Part model, mm, in its own coordinate system. A direction names the side the tool comes from. Coordinates: 2 decimals unless noted, no trailing zeros. One line per question, with ' | ' between items. Start each with the question number.
Autodesk Fusion 360 part; units mm, degrees
sketch "Sketch1" plane through (0, 0, 0) normal (0, 1, 0) x (1, 0, 0)
  circle A0 centre (0, 0) radius 57.5
  line L0 (36, -36) -> (-36, -36) construction
  line L1 (-36, -36) -> (-36, 36) construction
  line L2 (-36, 36) -> (36, 36) construction
  line L3 (36, 36) -> (36, -36) construction
  line L4 (36, -36) -> (-36, 36) construction
  line L5 (-36, -36) -> (36, 36) construction
  circle A1 centre (0, 0) radius 43
  circle A2 centre (-36, 36) radius 2
  circle A3 centre (36, 36) radius 2
  circle A4 centre (36, -36) radius 2
  circle A5 centre (-36, -36) radius 2
  circle A6 centre (-36, -36) radius 2.875
  circle A7 centre (36, -36) radius 2.875
  circle A8 centre (36, 36) radius 2.875
  circle A9 centre (-36, 36) radius 2.875
  line L6 (52.5, 40.4773) -> (52.5, -51.7956) construction
  line L7 (67.5556, 30.3847) -> (52.5, 30.3847)
  line L8 (52.5, 30.3847) -> (52.5, -29.8632)
  line L9 (-46.2969, -51.75) -> (48.3967, -51.75)
  arc A10 (-25.0637, -51.75) -> (25.0637, -51.75) centre (0, 0) ccw
  dimension "d1" = 115
  dimension "d2" = 72
  dimension "d3" = 72
  dimension "d4" = 86
  dimension "d5" = 4
  dimension "d6" = 4
  dimension "d7" = 4
  dimension "d8" = 4
  dimension "d9" = 5.75
  dimension "d10" = 5.75
  dimension "d11" = 5.75
  dimension "d12" = 5.75
  dimension "d54" = 52.5
  dimension "d58" = 51.75
extrude "Extrude1" add sketch "Sketch1" along normal blind 4 contours A0 L9 A10 | A0 L8 L9 | A0 L8
extrude "Extrude3" add sketch "Sketch1" along normal blind 2 contours A1
sketch "Sketch2" plane through (0, 2, 0) normal (0, 1, 0) x (-1, 0, 0)
  circle A0 centre (0, 0) radius 43
  circle A1 centre (0, 0) radius 35 construction
  circle A2 centre (0, 0) radius 27.5 construction
  circle A3 centre (0, 0) radius 20 construction
  circle A4 centre (0, 0) radius 12.5 construction
  circle A5 centre (0, 0) radius 7.5 construction
  circle A6 centre (-0.2536, -34.9991) radius 3.5
  circle A7 centre (10.5741, -33.3645) radius 3.5
  circle A8 centre (20.3668, -28.4639) radius 3.5
  circle A9 centre (28.1658, -20.7771) radius 3.5
  circle A10 centre (33.2077, -11.0565) radius 3.5
  circle A11 centre (34.9991, -0.2536) radius 3.5
  circle A12 centre (33.3645, 10.5741) radius 3.5
  circle A13 centre (28.4639, 20.3668) radius 3.5
  circle A14 centre (20.7771, 28.1658) radius 3.5
  circle A15 centre (11.0565, 33.2077) radius 3.5
  circle A16 centre (0.2536, 34.9991) radius 3.5
  circle A17 centre (-10.5741, 33.3645) radius 3.5
  circle A18 centre (-20.3668, 28.4639) radius 3.5
  circle A19 centre (-28.1658, 20.7771) radius 3.5
  circle A20 centre (-33.2077, 11.0565) radius 3.5
  circle A21 centre (-34.9991, 0.2536) radius 3.5
  circle A22 centre (-33.3645, -10.5741) radius 3.5
  circle A23 centre (-28.4639, -20.3668) radius 3.5
  circle A24 centre (-20.7771, -28.1658) radius 3.5
  circle A25 centre (-11.0565, -33.2077) radius 3.5
  circle A26 centre (4.2963, -27.1623) radius 3.5
  circle A27 centre (12.4797, -24.5053) radius 3.5
  circle A28 centre (19.4414, -19.4495) radius 3.5
  circle A29 centre (24.5001, -12.4898) radius 3.5
  circle A30 centre (27.1605, -4.3076) radius 3.5
  circle A31 centre (27.1623, 4.2963) radius 3.5
  circle A32 centre (24.5053, 12.4797) radius 3.5
  circle A33 centre (19.4495, 19.4414) radius 3.5
  circle A34 centre (12.4898, 24.5001) radius 3.5
  circle A35 centre (4.3076, 27.1605) radius 3.5
  circle A36 centre (-4.2963, 27.1623) radius 3.5
  circle A37 centre (-12.4797, 24.5053) radius 3.5
  circle A38 centre (-19.4414, 19.4495) radius 3.5
  circle A39 centre (-24.5001, 12.4898) radius 3.5
  circle A40 centre (-27.1605, 4.3076) radius 3.5
  circle A41 centre (-27.1623, -4.2963) radius 3.5
  circle A42 centre (-24.5053, -12.4797) radius 3.5
  circle A43 centre (-19.4495, -19.4414) radius 3.5
  circle A44 centre (-12.4898, -24.5001) radius 3.5
  circle A45 centre (-4.3076, -27.1605) radius 3.5
  circle A46 centre (0.1335, -19.9996) radius 3.5
  circle A47 centre (11.8634, -16.1015) radius 3.5
  circle A48 centre (19.0619, -6.0533) radius 3.5
  circle A49 centre (18.9795, 6.3071) radius 3.5
  circle A50 centre (11.6475, 16.2584) radius 3.5
  circle A51 centre (-0.1335, 19.9996) radius 3.5
  circle A52 centre (-11.8634, 16.1015) radius 3.5
  circle A53 centre (-19.0619, 6.0533) radius 3.5
  circle A54 centre (-18.9795, -6.3071) radius 3.5
  circle A55 centre (-11.6475, -16.2584) radius 3.5
  circle A56 centre (4.3124, -11.7326) radius 3.5
  circle A57 centre (10.3851, -6.957) radius 3.5
  circle A58 centre (12.4909, 0.4758) radius 3.5
  circle A59 centre (9.8257, 7.7269) radius 3.5
  circle A60 centre (3.4074, 12.0266) radius 3.5
  circle A61 centre (-4.3124, 11.7326) radius 3.5
  circle A62 centre (-10.3851, 6.957) radius 3.5
  circle A63 centre (-12.4909, -0.4758) radius 3.5
  circle A64 centre (-9.8257, -7.7269) radius 3.5
  circle A65 centre (-3.4074, -12.0266) radius 3.5
  circle A66 centre (-0.0342, -5.0724) radius 2.5
  circle A67 centre (4.8135, -1.6) radius 2.5
  circle A68 centre (3.0092, 4.0835) radius 2.5
  circle A69 centre (-2.9538, 4.1238) radius 2.5
  circle A70 centre (-4.8347, -1.5349) radius 2.5
  dimension "d19" = 70
  dimension "d20" = 55
  dimension "d21" = 40
  dimension "d22" = 25
  dimension "d23" = 15
  dimension "d24" = 7
  dimension "d28" = 360
  dimension "d29" = 7
  dimension "d31" = 360
  dimension "d32" = 7
  dimension "d34" = 360
  dimension "d35" = 7
  dimension "d43" = 360
  dimension "d45" = 5
  dimension "d47" = 360
extrude "Extrude4" cut sketch "Sketch2" against normal up to surface (2 mm away) contours A6
extrude "Extrude5" cut sketch "Sketch2" against normal up to surface (2 mm away) contours A7 | A8 | A9 | A10 | A11 | A12 | A13 | A14 | A15 | A16 | A17 | A18 | A19 | A20 | A21 | A22 | A23 | A24 | A25 | A26 | A27 | A28 | A29 | A30 | A31 | A32 | A33 | A34 | A35 | A36 | A37 | A38 | A39 | A40 | A41 | A42 | A43 | A44 | A45 | A46 | A47 | A48 | A49 | A50 | A51 | A52 | A53 | A54 | A55 | A56 | A57 | A58 | A59 | A60 | A61 | A62 | A63 | A64 | A65 | A66 | A67 | A68 | A69 | A70
extrude "Extrude6" add sketch "Sketch1" against normal blind 2 from surface at 4 contours A6 | A7 | A8 | A9
chamfer "Chamfer1" distance 3 angle 45 1 edges at (-53.6088, 0, 20.7929)
extrude "Extrude7" cut sketch "Sketch1" along normal up to surface (4 mm away) contours A0 L8
extrude "Extrude8" cut sketch "Sketch1" along normal up to surface (4 mm away) contours A0 L9 A10
equation "d54 = ( d1 / 2 ) - 5 mm"
equation "d58 = ( d1 / 2 ) - 5.75 mm"
1) Wall check: line 1 along Z through (x, y) = (37.5, 1.7); line 2 along X through (y, z) = (1.8, 20); line 3 along Z through (x, y) = (38, 0.6). Give the ranges that are in metal, low to high. Write a range as [from, to].
2) Mould opens along X. For faces 4 (the cylindrical face through (-41.12, 3.49, -40.19)), 5 (the cylindrical face through (10.876, 1.014, -3.581)) say: +X half, -X half, draft (parallel to the pull), parting line (faces both ways), or undercut.
3) Band-saw the part on A-A on y = 1.3. Count the separate pieces of the cut face and the enclosed holes in it, then the cut area to 3 significant figures.
4) Pin check, flat tips, straight feed: pin 1 Ø9 at (x, z) = (33.21, 11.06) entering from +Y; pin 2 Ø4.5 at (x, z) = (-36, 36) entering from -Y. Stop position of each tip, or through.
5) Tool access for faces 1 (the cylindrical face through (5.066, 1.014, -30.577)), 2 (the cylindrical face through (-38.12, 0.99, 37.94)), 3 (the cylindrical face through (-5.598, 2.986, 42.634)): list every direction of +Z, -Z, +X, -X, +Y, -Y with a clear straight run to the whole face (end or side of a thin tool).
Values found:
1) line 1: [-41.86, -38.45], [-33.55, -2.19], [2.7, 33.55], [38.45, 41.86] | line 2: [-52.63, -31.94], [-24.98, -22.9], [-15.99, -3.37], [3.63, 15.98], [22.9, 24.75], [31.58, 52.5] | line 3: [-39.9, -38.07], [-33.93, -1.55], [2.05, 33.93], [38.07, 39.9]
2) face 4: parting line | face 5: undercut
3) separate pieces: 1 | enclosed holes: 69 | area: 7,070 mm²
4) pin 1: y = 2 | pin 2: y = 2
5) face 1: +Y, -Y | face 2: -Y | face 3: +Y
